Source: three-view drawing plus pictorial views. Frame: mm from the lowest corner of the part. A direction names the side the tool comes from. Give positions to 0.01 mm unless a question says otherwise; leave off trailing zeros. Write each loop counter-clockwise with the first axis right and the second up, starting at its lowest first coordinate (ties: lowest second). Pieces come first, ordered by that corner, then holes. Notation, with made-up numbers: M -5,71.25 L 38,71.25 A31 cw 38,107.25 Z; hole C 61,-8.75 d6. An arc over 180 degrees is marked long. Return JSON: item names as keys, results as strings.
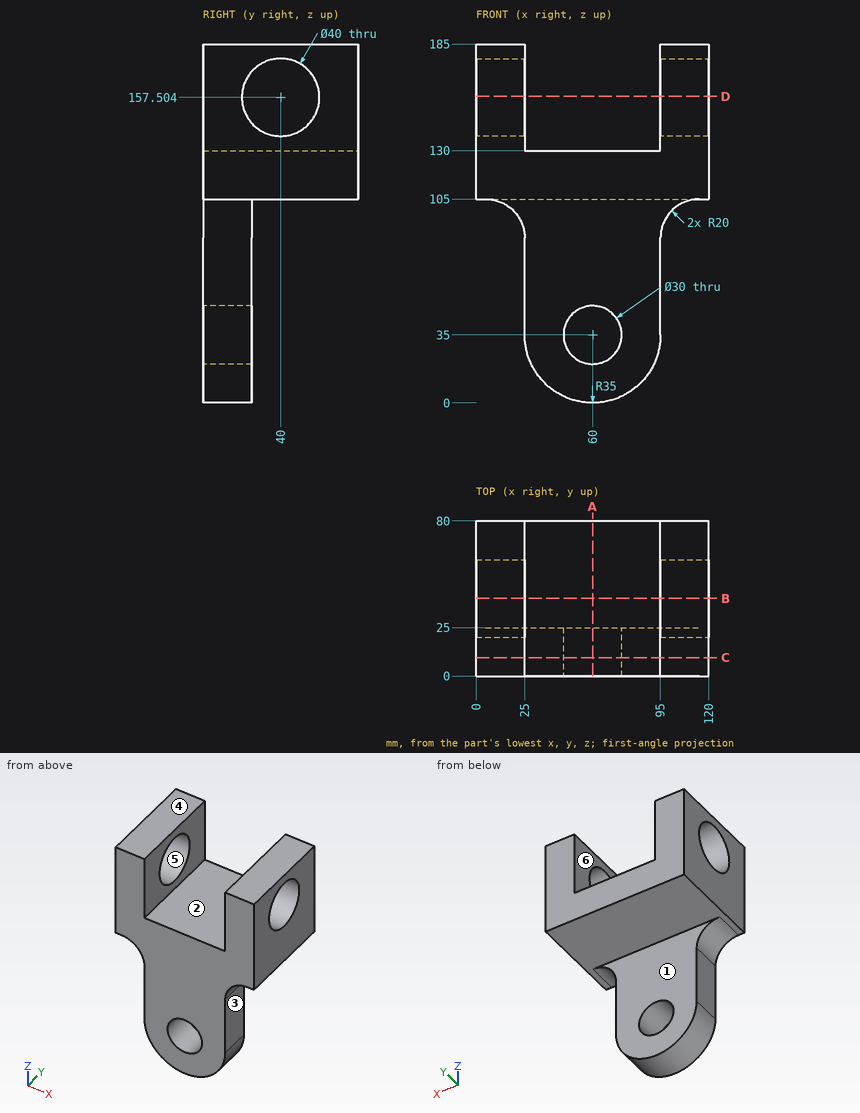
1) Draft query along Z for the marked faces 4, 5 and 6. Return one class per face: released by +Z, released by -Z, zero draft, split by the parting line, or undercut.
Numbers:
{"face 4": "released by +Z", "face 5": "undercut", "face 6": "zero draft"}
2) Line query: line 1 (X direction, y = 14.5, z = 164); line 2 (Y direction, x = 73, z = 49.5); line 3 (Z direction, x = 32, y = 76.5). Output: solid intervals per line, ascending. Write a range as [from, to].
Numbers:
{"line 1": "x = [0, 25], [95, 120]", "line 2": "y = [0, 25]", "line 3": "z = [105, 130]"}
3) Set-up query: the marked faces 1, 2 and 3. Return all of +Z, -Z, +X, -X, +Y, -Y with unobstructed straight access to the full face (end or side cutting, diameter ignored); none if empty.
Numbers:
{"face 1": "-Z, +X, -X, +Y", "face 2": "+Z, +Y, -Y", "face 3": "-Z, +X, +Y, -Y"}
4) Cut plane B-B, the plane y = 40. Return the cut outline in (x, z), then the cut area to 3 significant figures.
Numbers:
{"outline": "M 0,105 L 120,105 L 120,137.5 L 95,137.5 L 95,130 L 25,130 L 25,137.5 L 0,137.5 Z; M 0,177.5 L 25,177.5 L 25,185 L 0,185 Z; M 95,177.5 L 120,177.5 L 120,185 L 95,185 Z", "area": "3,750 mm²"}
5) Cut plane A-A, the plane x = 60. Return the cut outline in (y, z), then the cut area to 4 significant figures.
Numbers:
{"outline": "M 0,0 L 25,0 L 25,20 L 0,20 Z; M 0,50 L 25,50 L 25,105 L 80,105 L 80,130 L 0,130 Z", "area": "3,875 mm²"}
6) Cut plane C-C, the plane y = 9.5. Return the cut outline in (x, z), then the cut area to 3 significant figures.
Numbers:
{"outline": "M 0,105 L 5,105 A20 cw 25,85 L 25,35 A35 ccw 95,35 L 95,85 A20 cw 115,105 L 120,105 L 120,185 L 95,185 L 95,130 L 25,130 L 25,185 L 0,185 Z; hole C 60,35 d30", "area": "12,000 mm²"}
7) Contact query for flat-ended pins moving along their axis: pin 1 Ø6 at (y, z) = (43.5, 140) entering from +X; pin 2 Ø3 at (x, y) = (26.5, 43.5) entering from -Z; pin 3 Ø2 at (y, z) = (21, 28) entering from +X; pin 4 Ø20 at (y, z) = (14, 52.5) entering from -X. Output: stop coordinate, or through.
Numbers:
{"pin 1": "stops at x = 120", "pin 2": "stops at z = 105", "pin 3": "stops at x = 94.48", "pin 4": "stops at x = 25"}
8) Cut plane D-D, the plane z = 158. Return the cut outline in (x, y).
Numbers:
{"outline": "M 0,0 L 25,0 L 25,20.01 L 0,20.01 Z; M 0,59.99 L 25,59.99 L 25,80 L 0,80 Z; M 95,0 L 120,0 L 120,20.01 L 95,20.01 Z; M 95,59.99 L 120,59.99 L 120,80 L 95,80 Z"}
